The listing builds one solid part. Answer for the finished solid, in the listing's coordinates (mm). Give positions to 0.01 mm unless a question says otherwise; leave off trailing zeros. Loops run counter-clockwise (first coordinate to the right, second up) from the corner with the lowest first, then second, coordinate; pieces in that order, holes last. Notation, with made-up numbers: M 59.5,-37 L 66.5,-37 A15 ccw 66.5,-16 Z; hole C 1.5,5 d11. An arc over 180 degrees is marked long. Return JSON: item names as keys, results as strings.
from build123d import *

# Parameters (mm, degrees)
F1_DEPTH = 7.62
F2_R     = 5.08
F3_R     = 1.27
F4_DEPTH = 25.4


with BuildPart() as f1:
    # F0 (on Top) → F1 (new body)
    with BuildSketch(Plane.XY):
        with BuildLine():
            Line((44.45, 31.75), (-44.45, 31.75))
            ThreePointArc((-44.45, 31.75), (-46.3098719395, 27.2598719395), (-50.8, 25.4))
            Line((-50.8, 25.4), (-50.8, -25.4))
            ThreePointArc((-50.8, -25.4), (-46.3098719395, -27.2598719395), (-44.45, -31.75))
            Line((-44.45, -31.75), (44.45, -31.75))
            ThreePointArc((44.45, -31.75), (46.3098719395, -27.2598719395), (50.8, -25.4))
            Line((50.8, -25.4), (50.8, 25.4))
            ThreePointArc((50.8, 25.4), (46.3098719395, 27.2598719395), (44.45, 31.75))
        make_face()
    extrude(amount=F1_DEPTH)

    # F2
    f2_edges = [f1.edges().sort_by_distance(p)[0] for p in [
        (0, 31.75, 7.62),
        (-50.8, 0, 7.62),
        (50.8, 0, 7.62),
        (0, -31.75, 7.62),
        (-46.309872, 27.259872, 7.62),
        (-46.309872, -27.259872, 7.62),
        (46.309872, -27.259872, 7.62),
        (46.309872, 27.259872, 7.62),
    ]]
    fillet(f2_edges, radius=F2_R)

    # F3 (on face) → F4 (cut)
    with BuildSketch(Plane.XY.offset(7.62)):
        with Locations((-40.64, 0)):
            Circle(F3_R)
        with Locations((40.64, 0)):
            Circle(F3_R)
    extrude(amount=-F4_DEPTH, mode=Mode.SUBTRACT)


solid = f1.part
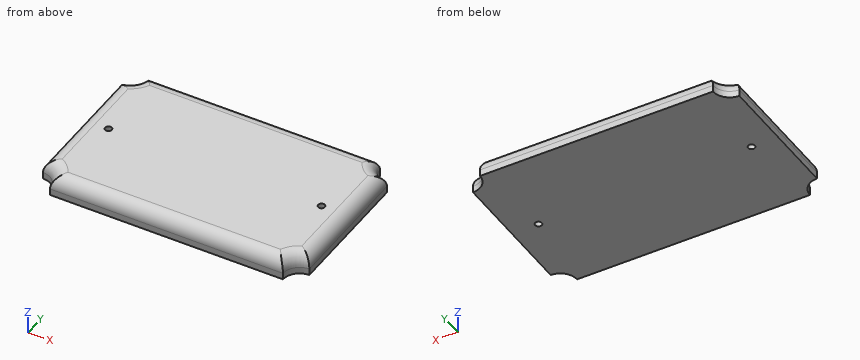
(1) Given pin 1 (3 mm diameter, centred on y = 18, z = 6, fed in from +X); pin 2 (2 mm diameter, centred on x = 26, z = 4, fed in from -Y); pin 3 (1.5 mm diameter, centred on y = 13.5, z = 4.5, fed in from -X); pin 4 (2 mm diameter, centred on x = -40.64, y = 0, fed in from -Z), each flat-ended and moving along its own axis, determine where each tip first touches the part or whether it passes through.
Values follow:
{"pin 1": "x = 50.41", "pin 2": "y = -31.73", "pin 3": "x = -50.65", "pin 4": "through"}
(2) The part is cut by section A-A (y = 0). Determine the outline of the cut face in (x, z), and give its area (3 significant figures).
Values follow:
{"outline": "M -50.8,0 L -41.91,0 L -41.91,7.62 L -45.72,7.62 A5.08 ccw -50.8,2.54 Z; M -39.37,0 L 39.37,0 L 39.37,7.62 L -39.37,7.62 Z; M 41.91,0 L 50.8,0 L 50.8,2.54 A5.08 ccw 45.72,7.62 L 41.91,7.62 Z", "area": "724 mm²"}
(3) Straight lines are drawn through the part: line 1 along Y through (x, z) = (-40.64, 2); line 2 along Y through (x, z) = (-40.64, 5.75); line 3 along Y through (x, z) = (-45.5, 5). For each, find the intervals that lie inside material, in ascending order.
Values follow:
{"line 1": "-31.75 to -1.27, 1.27 to 31.75", "line 2": "-30.61 to -1.27, 1.27 to 30.61", "line 3": "-27.2 to 27.2"}
(4) The part is cut by section B-B (z = 1.5). Determine the outline of the cut face in (x, y), and give its area (3 significant figures).
Values follow:
{"outline": "M -50.8,-25.4 A6.35 cw -44.45,-31.75 L 44.45,-31.75 A6.35 cw 50.8,-25.4 L 50.8,25.4 A6.35 cw 44.45,31.75 L -44.45,31.75 A6.35 cw -50.8,25.4 Z; hole C -40.64,0 d2.54; hole C 40.64,0 d2.54", "area": "6,310 mm²"}
(5) The part is cut by section C-C (x = -13.5). Determine the outline of the cut face in (y, z), and give its area (3 significant figures).
Values follow:
{"outline": "M -31.75,0 L 31.75,0 L 31.75,2.54 A5.08 ccw 26.67,7.62 L -26.67,7.62 A5.08 ccw -31.75,2.54 Z", "area": "473 mm²"}
